Check sheet for the modelled part. Datum: model origin and axes. Units: mm. A direction names the side the tool comes from. Coordinates: 2 decimals unless noted, no trailing zeros. Loops run counter-clockwise (first coordinate to the right, second up) from the corner with the lowest first, then second, coordinate; pieces in that order, holes last.
from build123d import *

# Parameters (mm, degrees)
ESQUISSE2_R        = 3.25
BOSS_EXTRU_1_DEPTH = 3
CONG_1_R           = 5


with BuildPart() as part:
    # Esquisse2 → Boss.-Extru.1 (new body)
    with BuildSketch(Plane.XY):
        Polygon((109.208492459, 1.901473412), (37.208492459, 1.901473412), (37.208492459, -43.098526588), (55.708492459, -43.098526588), (55.708492459, -58.098526588), (90.708492459, -58.098526588), (90.708492459, -43.098526588), (109.208492459, -43.098526588), align=None)
        with Locations((103.208492459, -4.098526588)):
            Circle(ESQUISSE2_R, mode=Mode.SUBTRACT)
        with Locations((103.208492459, -38.098526588)):
            Circle(ESQUISSE2_R, mode=Mode.SUBTRACT)
        with Locations((43.208492459, -38.098526588)):
            Circle(ESQUISSE2_R, mode=Mode.SUBTRACT)
        with Locations((43.208492459, -4.098526588)):
            Circle(ESQUISSE2_R, mode=Mode.SUBTRACT)
        with Locations((43.208492459, -21.098526588)):
            Circle(ESQUISSE2_R, mode=Mode.SUBTRACT)
        with Locations((103.208492459, -21.098526588)):
            Circle(ESQUISSE2_R, mode=Mode.SUBTRACT)
    extrude(amount=BOSS_EXTRU_1_DEPTH)

    # Congé1
    cong_1_edges = [part.edges().sort_by_distance(p)[0] for p in [
        (109.208492459, -43.098526588, 1.5),
        (90.708492459, -43.098526588, 1.5),
        (90.708492459, -58.098526588, 1.5),
        (55.708492459, -58.098526588, 1.5),
        (55.708492459, -43.098526588, 1.5),
        (37.208492459, -43.098526588, 1.5),
        (37.208492459, 1.901473412, 1.5),
        (109.208492459, 1.901473412, 1.5),
    ]]
    fillet(cong_1_edges, radius=CONG_1_R)


solid = part.part
(1) Set-up check for faces 4 (the face through (107.7, 0.48, 1.52)), 5 (the face through (90.708, -51, 1)): record each of +Z, -Z, +X, -X, +Y, -Y from which the full face is reachable in a straight line by a thin tool's end or side.
(2) Gauge pin test, flat ends, axial feed: P1, Ø6, axis at x = 43.21, y = -4.1, coming from the +Z side; P2, Ø0.9, axis at x = 45.5, z = 1.5, coming from the -Y side; P3, Ø1.5, axis at y = -51.5, z = 2, coming from the +X side. Record the tip position at first contact, or that the pin passes through.
(3) Section check C-C, the plane y = -51.5. Enter the section's corners in (x, z).
(4) Draft check along Y on faces 1 (the face through (40.63, -23.08, 1.48)), 2 (the face through (46, -43.099, 1)), 3 (the face through (55.708, -51, 1)). Enter one of: pulls with the +Y half, pulls with the -Y half, needs draft (parallel to the pull), parting line crosses it, or undercut.
(5) Section check B-B, the plane x = 48. Enter the section's corners in (y, z).
(6) Scan lines: line 1 along X through (y, z) = (-38, 2.6); line 2 along X through (y, z) = (-39, 1.2); line 3 along Y through (x, z) = (105, 1.5). Record each from-to range of solid material in increasing order.
(7) Section check A-A, the plane z = 1.45. Enter the section's corners in (x, y).
Determined:
1. face 4: +Z, -Z, +X, +Y
1. face 5: +Z, -Z, +X, -Y
2. P1: passes through
2. P2: stops at y = -43.1
2. P3: stops at x = 90.71
3. outline: (55.71, 0) - (90.71, 0) - (90.71, 3) - (55.71, 3) - close
4. face 1: undercut
4. face 2: pulls with the -Y half
4. face 3: needs draft
5. outline: (-43.1, 0) - (1.9, 0) - (1.9, 3) - (-43.1, 3) - close
6. line 1: x = 37.21 to 39.96, 46.46 to 99.96, 106.46 to 109.21
6. line 2: x = 37.29 to 40.09, 46.33 to 100.09, 106.33 to 109.13
6. line 3: y = -43.04 to -40.81, -35.39 to -23.81, -18.39 to -6.81, -1.39 to 1.84
7. outline: (37.21, -38.1) arc R5 ccw to (42.21, -43.1) - (50.71, -43.1) arc R5 cw to (55.71, -48.1) - (55.71, -53.1) arc R5 ccw to (60.71, -58.1) - (85.71, -58.1) arc R5 ccw to (90.71, -53.1) - (90.71, -48.1) arc R5 cw to (95.71, -43.1) - (104.21, -43.1) arc R5 ccw to (109.21, -38.1) - (109.21, -3.1) arc R5 ccw to (104.21, 1.9) - (42.21, 1.9) arc R5 ccw to (37.21, -3.1) - close; hole circle Ø6.5 at (43.21, -38.1); hole circle Ø6.5 at (43.21, -21.1); hole circle Ø6.5 at (43.21, -4.1); hole circle Ø6.5 at (103.21, -38.1); hole circle Ø6.5 at (103.21, -21.1); hole circle Ø6.5 at (103.21, -4.1)
